```python
from build123d import *

# Parameters (mm, degrees)
SKETCH_1_R           = 75
SKETCH_1_R_2         = 5
SKETCH_1_R_3         = 12.427488399
EXTRUDE_1_DEPTH      = 30
SKETCH_2_R           = 5
EXTRUDE_2_DEPTH      = 30
EXTRUDE_2_DEPTH_BACK = 60


with BuildPart() as part:
    # 草图1 → 凸台-拉伸1 (new body)
    with BuildSketch(Plane.XY):
        Circle(SKETCH_1_R)
        Circle(SKETCH_1_R_2, mode=Mode.SUBTRACT)
        with Locations((-30.195035009, 37.625475503)):
            Circle(SKETCH_1_R_3, mode=Mode.SUBTRACT)
    extrude(amount=EXTRUDE_1_DEPTH)

    # 草图2 → 凸台-拉伸2 (add, two sides)
    with BuildSketch(Plane.XY.offset(30)) as extrude_2_sk:
        Circle(SKETCH_2_R)
    extrude(amount=EXTRUDE_2_DEPTH)
    extrude(extrude_2_sk.sketch, amount=-EXTRUDE_2_DEPTH_BACK)


solid = part.part
```
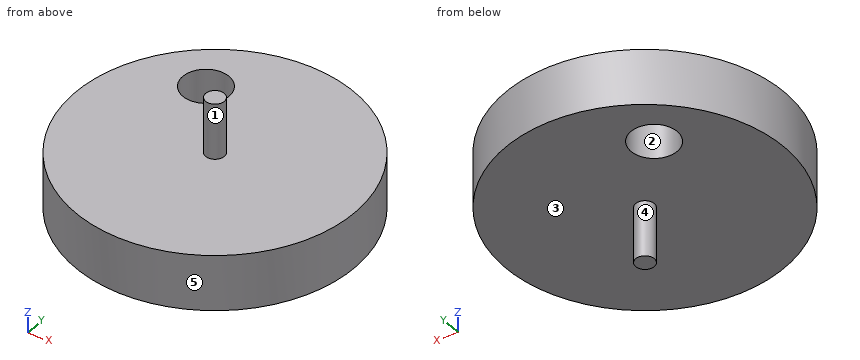
Could you check a few things on this model? Use its own coordinates, in mm. Face numbers are marked on the shaded views. A direction names the side the tool comes from. Round coordinates to 2 decimals unless told otherwise and drop trailing zeros. Write each loop counter-clockwise with the first axis right and the second up, starting at its lowest first coordinate (ties: lowest second). Pieces come first, ordered by that corner, then holes.
(1) Which directions (+Z, -Z, +X, -X, +Y, -Y) give clear straight access to the entire face, cutting with the end or side of a thin tool? Please do the marked faces 4 and 5.
Findings below:
face 4: -Z
face 5: +Z, -Z
(2) Suppose I cut it at B-B on y = 0. Write out the boundary of the cut face in (x, z), and give its area (3 significant figures).
Findings below:
outline: (-75, 0) - (-5, 0) - (-5, -30) - (5, -30) - (5, 0) - (75, 0) - (75, 30) - (5, 30) - (5, 60) - (-5, 60) - (-5, 30) - (-75, 30) - close
area: 5,100 mm2
(3) If I drill on probe 1 along Z at (x, y) = (-45, -15); probe 2 along Y at (x, z) = (-27, 13); probe 3 along X at (y, z) = (-2, 3), over which ranges is the centre line in solid material (lowest first)?
Findings below:
probe 1: z = 0 to 30
probe 2: y = -69.97 to 25.62, 49.64 to 69.97
probe 3: x = -74.97 to 74.97
(4) Thinking about a two-plate mould opening in X: for the marked faces 1, 2 and 3, which applies, +X half, -X half, draft (parallel to the pull), parting line (faces both ways), or undercut?
Findings below:
face 1: parting line
face 2: undercut
face 3: draft
(5) Suppose I cut it at A-A on x = -32. Write out the boundary of the cut face in (y, z), and give its area (3 significant figures).
Findings below:
outline: (-67.83, 0) - (25.33, 0) - (25.33, 30) - (-67.83, 30) - close; (49.92, 0) - (67.83, 0) - (67.83, 30) - (49.92, 30) - close
area: 3,330 mm2
(6) For pin 1 (12 mm diameter, centred on x = -25.5, z = 20.5, fed in from -Y); pin 2 (1.5 mm diameter, centred on x = 2.5, z = -11, fed in from -Y); pin 3 (4 mm diameter, centred on y = -31, z = 24, fed in from +X), each with a flat end and sliding along its axis, tell me the tip position at first contact or that it passes through.
Findings below:
pin 1: stops at y = -72.42
pin 2: stops at y = -4.68
pin 3: stops at x = 69.17
(7) Suppose I cut it at D-D on z = 3. Write out the boundary of the cut face in (x, y), and give its area (3 significant figures).
Findings below:
outline: circle Ø150 at (0, 0); hole circle Ø24.85 at (-30.2, 37.63)
area: 17,200 mm2
